from build123d import *

# Parameters (mm, degrees)
ESQUISSE4_W                                      = 275
ESQUISSE4_H                                      = 157
BOSS_EXTRU_2_DEPTH                               = 4
FRAISAGE_POUR_VIS_T_TE_FRAIS_E_M42_AT_COUNT      = 2
FRAISAGE_POUR_VIS_T_TE_FRAIS_E_M42_AT_PITCH      = 235.512207752
FRAISAGE_POUR_VIS_T_TE_FRAIS_E_M42_2_COUNT       = 2
FRAISAGE_POUR_VIS_T_TE_FRAIS_E_M42_2_PITCH       = 229
FRAISAGE_POUR_VIS_T_TE_FRAIS_E_M42_3_COUNT       = 2
FRAISAGE_POUR_VIS_T_TE_FRAIS_E_M42_3_PITCH       = 55
CHAMBRAGE_POUR_VIS_T_TE_RONDE_6_PANS_D           = 6.6
CHAMBRAGE_POUR_VIS_T_TE_RONDE_6_PANS_CBORE_D     = 11.5
CHAMBRAGE_POUR_VIS_T_TE_RONDE_6_PANS_CBORE_DEPTH = 2


with BuildPart() as part:
    # Esquisse4 → Boss.-Extru.2 (new body)
    with BuildSketch(Plane.XY):
        Rectangle(ESQUISSE4_W, ESQUISSE4_H)
    extrude(amount=BOSS_EXTRU_2_DEPTH)

    # Esquisse6 → Fraisage pour vis à tête fraisée M42 (revolve, cut)
    with BuildSketch(Plane(origin=(-114.5, -21, 0), x_dir=(0, 1, 0), z_dir=(1, 0, 0))):
        Polygon((0, 0), (0, 4), (2.25, 4), (2.25, 2.45), (4.7, 0), align=None)
    fraisage_pour_vis_t_te_frais_e_m42 = revolve(axis=Axis((-114.5, -21, -6.35), (0, 0, 1)), mode=Mode.SUBTRACT)

    # Fraisage pour vis à tête fraisée M42 at: Fraisage pour vis à tête fraisée M42 ×2
    with Locations(*[Vector(0.972348747, 0.233533542, 0) * (i * FRAISAGE_POUR_VIS_T_TE_FRAIS_E_M42_AT_PITCH) for i in range(1, FRAISAGE_POUR_VIS_T_TE_FRAIS_E_M42_AT_COUNT)]):
        add(fraisage_pour_vis_t_te_frais_e_m42, mode=Mode.SUBTRACT)

    # Fraisage pour vis _ t_te frais_e M42 2: Fraisage pour vis à tête fraisée M42 ×2
    with Locations(*[(i * FRAISAGE_POUR_VIS_T_TE_FRAIS_E_M42_2_PITCH, 0, 0) for i in range(1, FRAISAGE_POUR_VIS_T_TE_FRAIS_E_M42_2_COUNT)]):
        add(fraisage_pour_vis_t_te_frais_e_m42, mode=Mode.SUBTRACT)

    # Fraisage pour vis _ t_te frais_e M42 3: Fraisage pour vis à tête fraisée M42 ×2
    with Locations(*[(0, i * FRAISAGE_POUR_VIS_T_TE_FRAIS_E_M42_3_PITCH, 0) for i in range(1, FRAISAGE_POUR_VIS_T_TE_FRAIS_E_M42_3_COUNT)]):
        add(fraisage_pour_vis_t_te_frais_e_m42, mode=Mode.SUBTRACT)

    # Chambrage pour Vis à tête ronde à 6 pans creux M61 (through all)
    with Locations(Plane.XY.offset(4)):
        with Locations((128.5, -69.5), (-128.5, -69.5), (-128.5, 69.5), (128.5, 69.5)):
            CounterBoreHole(CHAMBRAGE_POUR_VIS_T_TE_RONDE_6_PANS_D / 2, CHAMBRAGE_POUR_VIS_T_TE_RONDE_6_PANS_CBORE_D / 2, CHAMBRAGE_POUR_VIS_T_TE_RONDE_6_PANS_CBORE_DEPTH)


solid = part.part
Part model, mm, in its own coordinate system. A direction names the side the tool comes from. Coordinates: 2 decimals unless noted, no trailing zeros. Loops run counter-clockwise (first coordinate to the right, second up) from the corner with the lowest first, then second, coordinate; pieces in that order, holes last. Notation, with made-up numbers: (81, -39.5) - (120, -39.5) arc R14 cw to (120, -32.5) - close; hole circle Ø3 at (4, -5). An arc over 180 degrees is marked (long way). Write each question's results on one line, items separated by ' | '. Start each with the question number.
Q1. Which spindle directions (+Z, -Z, +X, -X, +Y, -Y) get a long thin tool onto all of the face, cutting with end or side? Do faces 3 (the cylindrical face through (130.93, -67.27, 0.99)), 4 (the cylindrical face through (133.984, 71.227, 3.014)). Say none if no direction does.
Q2. Slice it at B-B on y = -69.5. Give the cut face in (x, z).
Q3. Slice it at A-A on x = -128.5. Give the cut face in (y, z), and give its area (3 significant figures).
Q4. Two-plate mould, pull along X, no slides. Class faces 1 (the flat face through (-2, 1, 0)), 2 (the conical face through (112.12, 33.69, 2.3)): +X half, -X half, draft (parallel to the pull), parting line (faces both ways), or undercut.
Q5. Probe line 1 along Y through (x, z) = (-128.5, 2.8); line 2 along Y through (x, z) = (-114.5, 3.2); line 3 along X through (y, z) = (70.5, 1.2). List the from-to ranges inside material, lowest first.
Q6. Drop flat-ended pins along their axis: pin 1 Ø6 at (x, y) = (-114.5, -21) entering from -Z; pin 2 Ø7 at (x, y) = (-114.5, 34) entering from -Z; pin 3 Ø6 at (x, y) = (-130.5, 71) entering from +Z. Give the stop position or say it passes through.
Answer:
1) face 3: +Z, -Z | face 4: +Z
2) outline: (-137.5, 0) - (-131.8, 0) - (-131.8, 2) - (-134.25, 2) - (-134.25, 4) - (-137.5, 4) - close; (-125.2, 0) - (125.2, 0) - (125.2, 2) - (122.75, 2) - (122.75, 4) - (-122.75, 4) - (-122.75, 2) - (-125.2, 2) - close; (131.8, 0) - (137.5, 0) - (137.5, 4) - (134.25, 4) - (134.25, 2) - (131.8, 2) - close
3) outline: (-78.5, 0) - (-72.8, 0) - (-72.8, 2) - (-75.25, 2) - (-75.25, 4) - (-78.5, 4) - close; (-66.2, 0) - (66.2, 0) - (66.2, 2) - (63.75, 2) - (63.75, 4) - (-63.75, 4) - (-63.75, 2) - (-66.2, 2) - close; (72.8, 0) - (78.5, 0) - (78.5, 4) - (75.25, 4) - (75.25, 2) - (72.8, 2) - close | area: 556 mm2
4) face 1: draft | face 2: undercut
5) line 1: y = -78.5 to -75.25, -63.75 to 63.75, 75.25 to 78.5 | line 2: y = -78.5 to -23.25, -18.75 to 31.75, 36.25 to 78.5 | line 3: x = -137.5 to -131.64, -125.36 to 125.36, 131.64 to 137.5
6) pin 1: stops at z = 1.7 | pin 2: stops at z = 1.2 | pin 3: stops at z = 2
